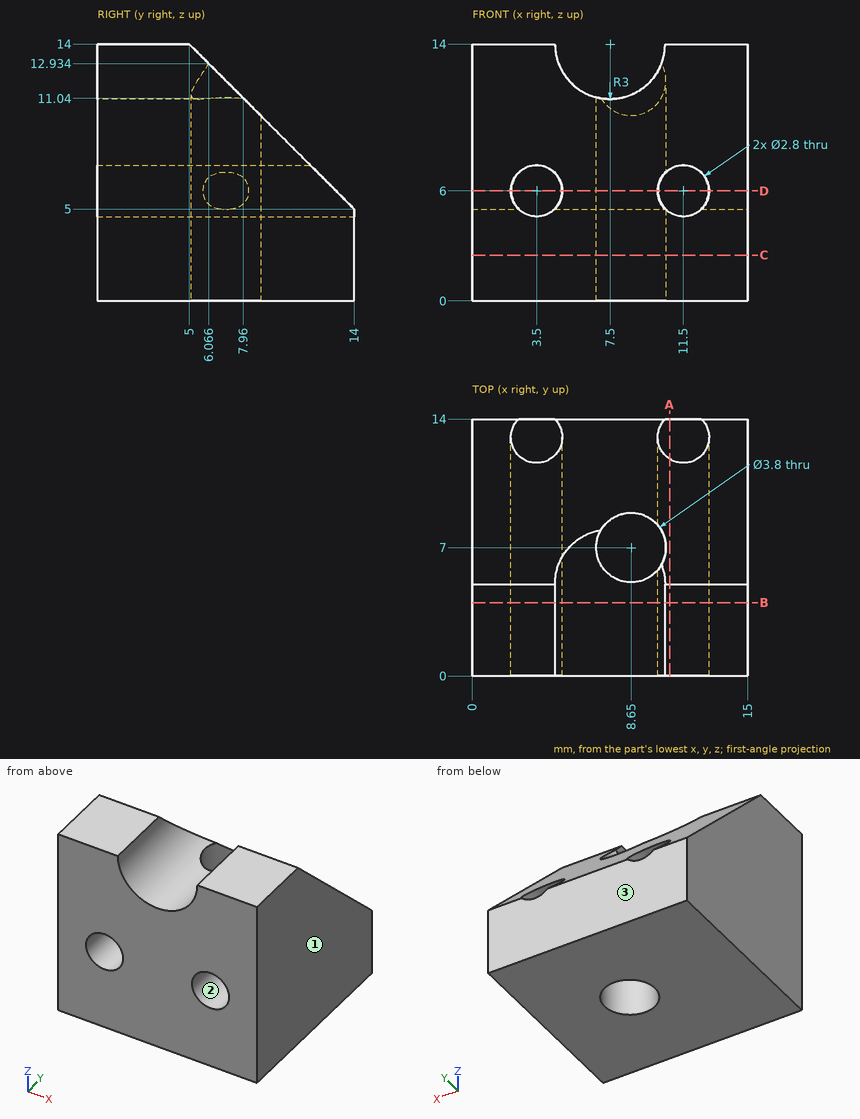
For this review, use the dimensioned drawing (mm, ordinates from the lowest corner) and the shaded views. Round coordinates to 2 decimals unless told otherwise and drop trailing zeros. Write each loop counter-clockwise with the first axis right and the second up, starting at its lowest first coordinate (ties: lowest second). Pieces come first, ordered by that corner, then holes. Notation, with made-up numbers: (33, 51) - (68, 51) arc R8 cw to (68, 59) - close; hole circle Ø3 at (70.25, -5). An arc over 180 degrees is marked (long way). Answer as a JSON object with one key per item and string values.
1. We need section D-D on z = 6. Give the boundary of the cut face in (x, y).
Response values:
{"outline": "(0, 0) - (2.1, 0) - (2.1, 13) - (0, 13) - close; (4.9, 0) - (10.1, 0) - (10.1, 5.77) arc R1.9 cw (long way) to (10.1, 8.23) - (10.1, 13) - (4.9, 13) - close; (12.9, 0) - (15, 0) - (15, 13) - (12.9, 13) - close"}
2. We need section C-C on z = 2.5. Give the boundary of the cut face in (x, y), then the cut area to 3 significant figures.
Response values:
{"outline": "(0, 0) - (15, 0) - (15, 14) - (0, 14) - close; hole circle Ø3.8 at (8.65, 7)", "area": "199 mm2"}
3. To check wall thickness, follow line 1 along X through (y, z) = (11, 6); line 2 along Z through (x, y) = (11.5, 4.25); line 3 along Y through (x, z) = (7.75, 4.5). State the ranges of each line that lie inside material, in increasing order.
Response values:
{"line 1": "x = 0 to 2.1, 4.9 to 10.1, 12.9 to 15", "line 2": "z = 0 to 4.6, 7.4 to 14", "line 3": "y = 0 to 5.33, 8.67 to 14"}
4. We need section A-A on x = 10.75. Give the boundary of the cut face in (y, z).
Response values:
{"outline": "(0, 0) - (14, 0) - (14, 4.82) - (0, 4.82) - close; (0, 7.18) - (11.82, 7.18) - (5, 14) - (0, 14) - close"}
5. We need section B-B on y = 4. Give the boundary of the cut face in (x, z).
Response values:
{"outline": "(0, 0) - (15, 0) - (15, 14) - (10.5, 14) arc R3 cw to (4.5, 14) - (0, 14) - close; hole circle Ø2.8 at (3.5, 6); hole circle Ø2.8 at (11.5, 6)"}
6. For pin 1 Ø5 at (x, z) = (8.5, 11) entering from +Y; pin 2 Ø3.5 at (x, y) = (8.65, 7) entering from -Z, all flat-tipped, find the tip position at first contact; note any pin that passes through.
Response values:
{"pin 1": "stops at y = 10.5", "pin 2": "passes through"}
7. Draft analysis for pull direction X (two halves, no side actions). For the marked faces 1, 2 and 3, state which applies: +X half, -X half, draft (parallel to the pull), parting line (faces both ways), or undercut.
Response values:
{"face 1": "+X half", "face 2": "undercut", "face 3": "draft"}
